```python
from build123d import *

# Parameters (mm, degrees)
SKETCH_W        = 150
SKETCH_H        = 135
PAD_DEPTH       = 15
SKETCH001_W     = 17
SKETCH001_H     = 30
PAD001_DEPTH    = 15
SKETCH002_W     = 150
SKETCH002_H     = 30
PAD002_DEPTH    = 150
SKETCH003_W     = 141.1
SKETCH003_H     = 25.2
POCKET_DEPTH    = 140
SKETCH004_W     = 15
SKETCH004_H     = 9
POCKET001_DEPTH = 10
SKETCH005_R     = 67.5
POCKET002_DEPTH = 30
SKETCH006_W     = 135.7
SKETCH006_H     = 100.1
POCKET003_DEPTH = 3.2
SKETCH007_R     = 3.1
PAD003_DEPTH    = 1.6
SKETCH008_R     = 1.4
POCKET004_DEPTH = 6
SKETCH009_R     = 1.55
PAD004_DEPTH    = 1.6
SKETCH010_W     = 135
SKETCH010_H     = 15
PAD005_DEPTH    = 10
SKETCH011_W     = 135
SKETCH011_H     = 15
PAD006_DEPTH    = 10
SKETCH012_W     = 7.6
SKETCH012_H     = 135
POCKET005_DEPTH = 11
SKETCH013_W     = 170
SKETCH013_H     = 15
PAD007_DEPTH    = 35
SKETCH014_W     = 150
SKETCH014_H     = 25
POCKET006_DEPTH = 11
SKETCH015_W     = 7.6
SKETCH015_H     = 26.2
POCKET007_DEPTH = 11
SKETCH016_W     = 167.6
SKETCH016_H     = 7.6
POCKET008_DEPTH = 10
SKETCH017_W     = 10
SKETCH017_H     = 10
POCKET009_DEPTH = 11
PAD008_DEPTH    = 11
SKETCH019_W     = 170
SKETCH019_H     = 15
PAD009_DEPTH    = 1.8
SKETCH020_W     = 171.8
SKETCH020_H     = 15
PAD010_DEPTH    = 1.8
SKETCH021_W     = 171.8
SKETCH021_H     = 15
PAD011_DEPTH    = 1.8


with BuildPart() as part:
    # Sketch → Pad (new body)
    with BuildSketch(Plane.XY):
        Rectangle(SKETCH_W, SKETCH_H)
    extrude(amount=PAD_DEPTH)

    # Sketch001 (on Face6 of Pad) → Pad001 (join)
    with BuildSketch(Plane.XY.offset(15)):
        with Locations((-66.5, -52.5)):
            Rectangle(SKETCH001_W, SKETCH001_H)
        with Locations((0, -52.5)):
            Rectangle(SKETCH001_W, SKETCH001_H)
        with Locations((66.5, -52.5)):
            Rectangle(SKETCH001_W, SKETCH001_H)
    extrude(amount=PAD001_DEPTH)

    # Sketch002 (on Face18 of Pad001) → Pad002 (join)
    with BuildSketch(Plane.XY.offset(30)):
        with Locations((0, -52.5)):
            Rectangle(SKETCH002_W, SKETCH002_H)
    extrude(amount=PAD002_DEPTH)

    # Sketch003 (on Face24 of Pad002) → Pocket (cut)
    with BuildSketch(Plane.XY.offset(180)):
        with Locations((0, -52.5)):
            Rectangle(SKETCH003_W, SKETCH003_H)
    extrude(amount=-POCKET_DEPTH, mode=Mode.SUBTRACT)

    # Sketch004 (on Face30 of Pocket) → Pocket001 (cut)
    with BuildSketch(Plane.XY.offset(40)):
        with Locations((-31.05, -52.4)):
            Rectangle(SKETCH004_W, SKETCH004_H)
    extrude(amount=-POCKET001_DEPTH, mode=Mode.SUBTRACT)

    # Sketch005 (on Face20 of Pocket001) → Pocket002 (cut)
    with BuildSketch(Plane.XZ.offset(67.5)):
        with Locations((0, 111)):
            Circle(SKETCH005_R)
    extrude(amount=-POCKET002_DEPTH, mode=Mode.SUBTRACT)

    # Sketch006 (on Face5 of Pocket002) → Pocket003 (cut)
    with BuildSketch(Plane.XY.offset(15)):
        with Locations((0, 17.45)):
            Rectangle(SKETCH006_W, SKETCH006_H)
    extrude(amount=-POCKET003_DEPTH, mode=Mode.SUBTRACT)

    # Sketch007 (on Face8 of Pocket003) → Pad003 (join)
    with BuildSketch(Plane.XY.offset(11.8)):
        with Locations((-62.15, 56.5)):
            Circle(SKETCH007_R)
        with Locations((-62.15, -26)):
            Circle(SKETCH007_R)
        with Locations((62.35, -26)):
            Circle(SKETCH007_R)
        with Locations((62.35, 56.5)):
            Circle(SKETCH007_R)
        with Locations((4.65, 14)):
            Circle(SKETCH007_R)
    extrude(amount=PAD003_DEPTH)

    # Sketch008 (on Face37 of Pad003) → Pocket004 (cut)
    with BuildSketch(Plane.XY.offset(13.4)):
        with Locations((-62.15, 56.5)):
            Circle(SKETCH008_R)
        with Locations((62.35, -26)):
            Circle(SKETCH008_R)
        with Locations((62.35, 56.5)):
            Circle(SKETCH008_R)
        with Locations((-62.15, -26)):
            Circle(SKETCH008_R)
    extrude(amount=-POCKET004_DEPTH, mode=Mode.SUBTRACT)

    # Sketch009 (on Face36 of Pocket004) → Pad004 (join)
    with BuildSketch(Plane.XY.offset(13.4)):
        with Locations((4.65, 14)):
            Circle(SKETCH009_R)
    extrude(amount=PAD004_DEPTH)

    # Sketch010 (on Face10 of Pad004) → Pad005 (join)
    with BuildSketch(Plane.YZ.offset(75)):
        with Locations((0, 7.5)):
            Rectangle(SKETCH010_W, SKETCH010_H)
    extrude(amount=PAD005_DEPTH)

    # Sketch011 (on Face1 of Pad005) → Pad006 (join)
    with BuildSketch(Plane(origin=(-75, 0, 0), x_dir=(0, -1, 0), z_dir=(-1, 0, 0))):
        with Locations((0, 7.5)):
            Rectangle(SKETCH011_W, SKETCH011_H)
    extrude(amount=PAD006_DEPTH)

    # Sketch012 (on Face14 of Pad006) → Pocket005 (cut)
    with BuildSketch(Plane.XY.offset(15)):
        with Locations((-80, 0)):
            Rectangle(SKETCH012_W, SKETCH012_H)
        with Locations((80, 0)):
            Rectangle(SKETCH012_W, SKETCH012_H)
    extrude(amount=-POCKET005_DEPTH, mode=Mode.SUBTRACT)

    # Sketch013 (on Face10 of Pocket005) → Pad007 (join)
    with BuildSketch(Plane.XZ.offset(67.5)):
        with Locations((0, 7.5)):
            Rectangle(SKETCH013_W, SKETCH013_H)
    extrude(amount=PAD007_DEPTH)

    # Sketch014 (on Face21 of Pad007) → Pocket006 (cut)
    with BuildSketch(Plane.XY.offset(15)):
        with Locations((0, -80)):
            Rectangle(SKETCH014_W, SKETCH014_H)
    extrude(amount=-POCKET006_DEPTH, mode=Mode.SUBTRACT)

    # Sketch015 (on Face42 of Pocket006) → Pocket007 (cut)
    with BuildSketch(Plane.XY.offset(15)):
        with Locations((-80, -80.6)):
            Rectangle(SKETCH015_W, SKETCH015_H)
        with Locations((80, -80.6)):
            Rectangle(SKETCH015_W, SKETCH015_H)
    extrude(amount=-POCKET007_DEPTH, mode=Mode.SUBTRACT)

    # Sketch016 (on Face42 of Pocket007) → Pocket008 (cut)
    with BuildSketch(Plane.XY.offset(15)):
        with Locations((0, -97.5)):
            Rectangle(SKETCH016_W, SKETCH016_H)
    extrude(amount=-POCKET008_DEPTH, mode=Mode.SUBTRACT)

    # Sketch017 (on Face42 of Pocket008) → Pocket009 (cut)
    with BuildSketch(Plane.XY.offset(15)):
        with Locations((-71.2, -88.7)):
            Rectangle(SKETCH017_W, SKETCH017_H)
        with Locations((71.2, -88.7)):
            Rectangle(SKETCH017_W, SKETCH017_H)
    extrude(amount=-POCKET009_DEPTH, mode=Mode.SUBTRACT)

    # Sketch018 (on Face80 of Pocket009) → Pad008 (join)
    with BuildSketch(Plane.XY.offset(4)):
        with BuildLine():
            ThreePointArc((66.2, -92.5), (72.42254, -89.92254), (75, -83.7))
            Line((75, -83.7), (76.2, -83.7))
            ThreePointArc((66.2, -93.7), (73.271068, -90.771068), (76.2, -83.7))
            Line((66.2, -93.7), (66.2, -92.5))
        make_face()
        with BuildLine():
            ThreePointArc((-75, -83.7), (-72.42254, -89.92254), (-66.2, -92.5))
            Line((-66.2, -93.7), (-66.2, -92.5))
            ThreePointArc((-76.2, -83.7), (-73.271068, -90.771068), (-66.2, -93.7))
            Line((-76.2, -83.7), (-75, -83.7))
        make_face()
    extrude(amount=PAD008_DEPTH)

    # Sketch019 (on Face17 of Pad008) → Pad009 (join)
    with BuildSketch(Plane(origin=(-85, 0, 0), x_dir=(0, -1, 0), z_dir=(-1, 0, 0))):
        with Locations((17.5, 7.5)):
            Rectangle(SKETCH019_W, SKETCH019_H)
    extrude(amount=PAD009_DEPTH)

    # Sketch020 (on Face40 of Pad009) → Pad010 (join)
    with BuildSketch(Plane.XZ.offset(102.5)):
        with Locations((-0.9, 7.5)):
            Rectangle(SKETCH020_W, SKETCH020_H)
    extrude(amount=PAD010_DEPTH)

    # Sketch021 (on Face39 of Pad010) → Pad011 (join)
    with BuildSketch(Plane.YZ.offset(85)):
        with Locations((-18.4, 7.5)):
            Rectangle(SKETCH021_W, SKETCH021_H)
    extrude(amount=PAD011_DEPTH)


solid = part.part
```
Part model, mm, in its own coordinate system. A direction names the side the tool comes from. Coordinates: 2 decimals unless noted, no trailing zeros. Write each loop counter-clockwise with the first axis right and the second up, starting at its lowest first coordinate (ties: lowest second). Pieces come first, ordered by that corner, then holes.
Item 1: Pin check, flat tips, straight feed: pin 1 (1.5 mm diameter, centred on y = -47.5, z = 62.5, fed in from +X); pin 2 (2 mm diameter, centred on x = -62.5, y = -26, fed in from +Z); pin 3 (6 mm diameter, centred on y = -45.5, z = 86, fed in from -X). Stop position of each tip, or through.
Item 2: Mould opens along Y. For faces 6 (the face through (-1, -104.3, 7)), 7 (the face through (-31, -56.9, 35)), 8 (the face through (76.2, -9, 10)) say: released by +Y, released by -Y, zero draft, split by the parting line, or undercut.
Item 3: Slice it at A-A (z = 37.5). Write the cut outline in (x, y), and give its area (4 significant figures).
Item 4: Slice it at B-B (x = -48.5). Count the separate pieces of the cut face and the enclosed holes in it, and give its area (3 significant figures).
Item 5: Probe line 1 (X direction, y = -59, z = 13); line 2 (Y direction, x = 62, z = 11); line 3 (Y direction, x = -64.5, z = 57.5). List the from-to ranges inside material, lowest first.
Item 6: Slice it at D-D (y = -11.5). Write the cut outline in (x, z), and give its area (3 significant figures).
Item 7: Which spindle directions (+Z, -Z, +X, -X, +Y, -Y) get a long thin tool onto all of the face, cutting with end or side? Do faces 1 (the face through (86.8, -20, 8)), 2 (the face through (-1, -93.7, 10)), 3 (the face through (-1, 67.5, 6)), 4 (the face through (-64, 57, 13.4)), 5 (the face through (8.5, -53, 22)). Say none if no direction does.
Item 8: Slice it at C-C (z = 111). Write the cut outline in (x, y), and give its area (3 significant figures).
Results found:
1. pin 1: stops at x = 75
1. pin 2: stops at z = 7.4
1. pin 3: stops at x = -75
2. face 6: released by -Y
2. face 7: undercut
2. face 8: zero draft
3. outline: (-75, -67.5) - (75, -67.5) - (75, -37.5) - (-75, -37.5) - close; hole (-38.55, -56.9) - (-23.55, -56.9) - (-23.55, -47.9) - (-38.55, -47.9) - close
3. area: 4,365 mm2
4. separate pieces: 4
4. enclosed holes: 0
4. area: 2,430 mm2
5. line 1: x = -86.8 to -83.8, -76.2 to 76.2, 83.8 to 86.8
5. line 2: y = -104.3 to -101.3, -93.7 to -92.5, -67.5 to -27.36, -24.64 to 55.14, 57.86 to 67.5
5. line 3: y = -67.5 to -65.1, -39.9 to -37.5
6. outline: (-86.8, 0) - (86.8, 0) - (86.8, 15) - (83.8, 15) - (83.8, 4) - (76.2, 4) - (76.2, 15) - (67.85, 15) - (67.85, 11.8) - (-67.85, 11.8) - (-67.85, 15) - (-76.2, 15) - (-76.2, 4) - (-83.8, 4) - (-83.8, 15) - (-86.8, 15) - close
6. area: 2,000 mm2
7. face 1: +Z, -Z, +X, +Y, -Y
7. face 2: +Z
7. face 3: +Z, -Z, +X, -X, +Y
7. face 4: +Z, +Y
7. face 5: +Y, -Y
8. outline: (-75, -67.5) - (-67.5, -67.5) - (-67.5, -65.1) - (-70.55, -65.1) - (-70.55, -39.9) - (-67.5, -39.9) - (-67.5, -37.5) - (-75, -37.5) - close; (67.5, -67.5) - (75, -67.5) - (75, -37.5) - (67.5, -37.5) - (67.5, -39.9) - (70.55, -39.9) - (70.55, -65.1) - (67.5, -65.1) - close
8. area: 296 mm2
